Geometry: see drawing. Coordinates: mm, zero at the bounding-box minimum. A direction names the side the tool comes from. Coordinates: 2 decimals unless noted, no trailing zeros. Write each loop counter-clockwise with the first axis right and the second up, starting at its lowest first coordinate (ties: lowest second). Pieces come first, ordered by that corner, then holes. Notation, with made-up numbers: M 15.5,-32.75 L 37.5,-32.75 A18 ccw 37.5,-17.75 Z; hole C -31.75,41.25 d5. An arc over 180 degrees is marked long. Write item = value, one per line. Start each with the question number.
1. Pin query (flat end, axial travel): pin 1 Ø3 at (y, z) = (11, 11.5) entering from +X; pin 2 Ø1.5 at (x, z) = (29, 9.5) entering from +Y; pin 3 Ø8 at (y, z) = (11, 11.5) entering from +X (1 decimal); pin 4 Ø1.5 at (x, y) = (38, 18.5) entering from +Z. Return the tip coordinate at first contact, or that it passes through.
2. Section query D-D (z = 7). Output: boundary loops of the cut face in (x, y) (1 decimal).
3. Line query: line 1 along X through (y, z) = (7.5, 1.75) (1 decimal); line 2 along X through (y, z) = (13.75, 14.5) (1 decimal); line 3 along Z through (x, y) = (27.55, 11). Output: solid intervals per line, ascending.
4. Section query C-C (x = 11). Output: boundary loops of the cut face in (y, z), then the cut area to 3 significant figures.
5. Pull-direction query (X, two-part tool) for the marked faces 1, 2, 3 and 4; classes: pulls with the +X half, pulls with the -X half, needs draft (parallel to the pull), parting line crosses it, or undercut.
6. Section query A-A (y = 5). Output: boundary loops of the cut face in (x, z) (1 decimal).
7. Access query for the marked faces 5, 6 and 7. Directions: +Z, -Z, +X, -X, +Y, -Y. A direction counts if a zero-diameter tool reaches every point of the face in a straight line with its end or side. Return the directions, or none.
8. Section query B-B (z = 17.5). Output: boundary loops of the cut face in (x, y) (1 decimal).
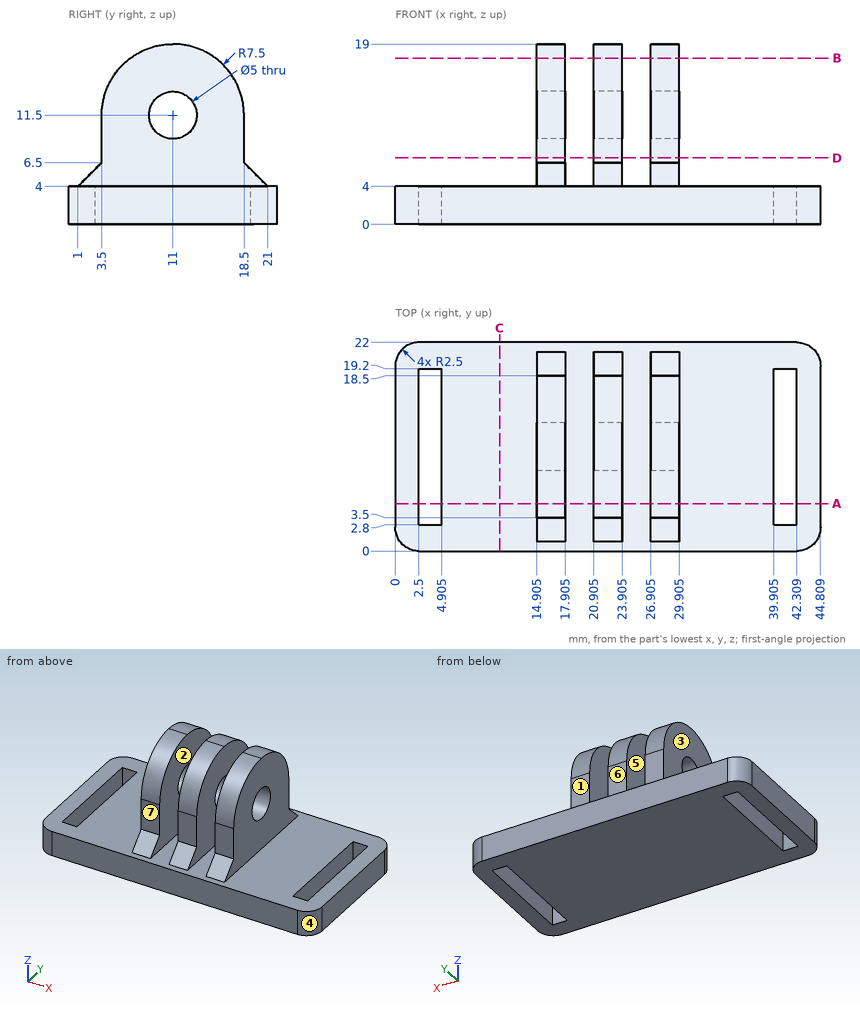
Results are:
q1.pin_1 = through
q1.pin_2 = 18.5
q1.pin_3 = 29.9
q1.pin_4 = 4
q2.outline = M 14.9,3.5 L 17.9,3.5 L 17.9,18.5 L 14.9,18.5 Z; M 20.9,3.5 L 23.9,3.5 L 23.9,18.5 L 20.9,18.5 Z; M 26.9,3.5 L 29.9,3.5 L 29.9,18.5 L 26.9,18.5 Z
q3.line_1 = 0 to 2.5, 4.9 to 39.9, 42.3 to 44.8
q3.line_2 = 14.9 to 17.9, 20.9 to 23.9, 26.9 to 29.9
q3.line_3 = 0 to 9, 14 to 19
q4.outline = M 0,0 L 22,0 L 22,4 L 0,4 Z
q4.area = 88.0 mm^2
q5.face_1 = needs draft
q5.face_2 = undercut
q5.face_3 = pulls with the -X half
q5.face_4 = pulls with the +X half
q6.outline = M 0,0 L 2.5,0 L 2.5,4 L 0,4 Z; M 4.9,0 L 39.9,0 L 39.9,4 L 29.9,4 L 29.9,16 L 26.9,16 L 26.9,4 L 23.9,4 L 23.9,16 L 20.9,16 L 20.9,4 L 17.9,4 L 17.9,16 L 14.9,16 L 14.9,4 L 4.9,4 Z; M 42.3,0 L 44.8,0 L 44.8,4 L 42.3,4 Z
q7.face_5 = +Z, +Y, -Y
q7.face_6 = +Z, +X, -X, +Y
q7.face_7 = +Z, +X, -X, -Y
q8.outline = M 14.9,6.5 L 17.9,6.5 L 17.9,15.5 L 14.9,15.5 Z; M 20.9,6.5 L 23.9,6.5 L 23.9,15.5 L 20.9,15.5 Z; M 26.9,6.5 L 29.9,6.5 L 29.9,15.5 L 26.9,15.5 Z
